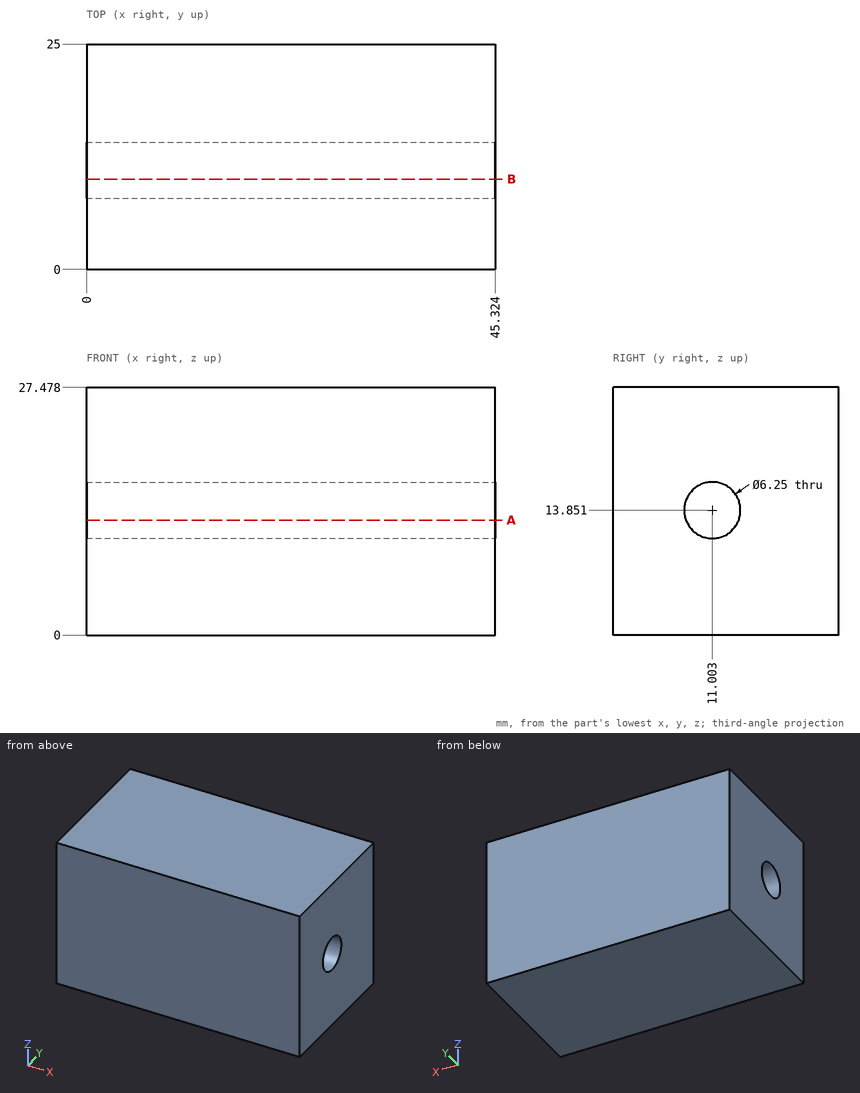
Geometry check sheet. Reference: drawing and pictorial views, mm from the part's lowest x, y, z. Give positions to 0.01 mm unless a question says otherwise; leave off trailing zeros. Order: outer loops, then holes, each group sorted by start corner. A loop starts at its lowest first (then second) coordinate and runs counter-clockwise, first axis right, second up. Notation, with made-up numbers: (15, -6) - (43, -6) arc R25 ccw to (43, 29) - close; hole circle Ø11 at (87.5, -11.5). An arc over 180 degrees is marked (long way). Answer as CSV lines item,"result". Start each with the question number.
Item 1: Material ranges on L1, parallel to Z at x = 41.5, y = 9.75 (1 decimal); L2, parallel to Z at x = 32, y = 11.75 (1 decimal), recorded low to high.
Item 2: Gauge pin test, flat end, axial feed: pin 1 (5.5 mm diameter, centred on y = 11, z = 13.85, fed in from -X). Record the tip position at first contact, or that the pin passes through.
Item 3: Section check B-B, the plane y = 10. Record the boundary of the cut face in (x, z), plus the area to 3 significant figures.
Item 4: Section check A-A, the plane z = 12.75. Record the boundary of the cut face in (x, y), plus the area to 3 significant figures.
Filled in:
1,L1,"0 to 11, 16.7 to 27.5"
1,L2,"0 to 10.8, 16.9 to 27.5"
2,pin 1,"through"
3,outline,"(0, 0) - (45.32, 0) - (45.32, 10.89) - (0, 10.89) - close; (0, 16.81) - (45.32, 16.81) - (45.32, 27.48) - (0, 27.48) - close"
3,area,"977 mm^2"
4,outline,"(0, 0) - (45.32, 0) - (45.32, 8.08) - (0, 8.08) - close; (0, 13.93) - (45.32, 13.93) - (45.32, 25) - (0, 25) - close"
4,area,"868 mm^2"
